Could you check a few things on this model? Use its own coordinates, in mm. Face numbers are marked on the shaded views. Coordinates: 2 decimals unless noted, no trailing zeros. Order: outer loops, then holes, each group sorted by start corner. A loop starts at its lowest first (then second) coordinate and runs counter-clockwise, first axis right, second up. Notation, with made-up numbers: M 60.5,16 L 102.5,16 A32 cw 102.5,52 Z; hole C 7.25,40.5 d9. An arc over 180 degrees is marked long. Write item = value, one per line. Start each with the question number.
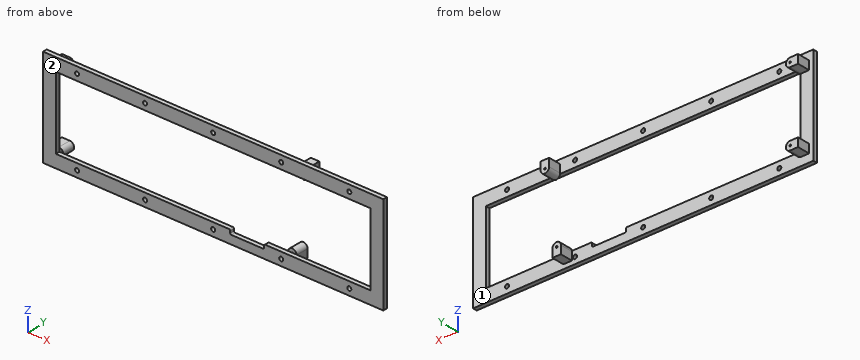
from build123d import *

# Parameters (mm, degrees)
SKETCH1_W           = 254
SKETCH1_H           = 72.69988
SKETCH1_R           = 1.5
BOSS_EXTRUDE1_DEPTH = 3.175
SKETCH1_7_R         = 0.635
BOSS_EXTRUDE2_DEPTH = 9.525


with BuildPart() as part:
    # Sketch1 → Boss-Extrude1 (new body)
    with BuildSketch(Plane(origin=(0, 0, 0), x_dir=(1, 0, 0), z_dir=(0, 1, 0))):
        with Locations((127, 36.34994)):
            Rectangle(SKETCH1_W, SKETCH1_H)
        with Locations(Location((177.8, 67.93738, 0), (0, 0, 270))):
            Circle(SKETCH1_R, mode=Mode.SUBTRACT)
        with Locations(Location((177.8, 4.7625, 0), (0, 0, 90))):
            Circle(SKETCH1_R, mode=Mode.SUBTRACT)
        with Locations(Location((228.6, 67.93738, 0), (0, 0, 270))):
            Circle(SKETCH1_R, mode=Mode.SUBTRACT)
        with Locations(Location((228.6, 4.7625, 0), (0, 0, 90))):
            Circle(SKETCH1_R, mode=Mode.SUBTRACT)
        with Locations(Location((127, 67.93738, 0), (0, 0, 270))):
            Circle(SKETCH1_R, mode=Mode.SUBTRACT)
        with Locations(Location((127, 4.7625, 0), (0, 0, 90))):
            Circle(SKETCH1_R, mode=Mode.SUBTRACT)
        with Locations(Location((25.4, 4.7625, 0), (0, 0, 270))):
            Circle(SKETCH1_R, mode=Mode.SUBTRACT)
        with Locations(Location((76.2, 4.7625, 0), (0, 0, 270))):
            Circle(SKETCH1_R, mode=Mode.SUBTRACT)
        with Locations(Location((25.4, 67.93738, 0), (0, 0, 90))):
            Circle(SKETCH1_R, mode=Mode.SUBTRACT)
        with Locations(Location((76.2, 67.93738, 0), (0, 0, 90))):
            Circle(SKETCH1_R, mode=Mode.SUBTRACT)
        with BuildLine():
            Line((244.475, 63.17488), (244.475, 9.525))
            Line((244.475, 9.525), (9.525, 9.525))
            Line((9.525, 9.525), (9.525, 63.17488))
            Line((9.525, 63.17488), (138.90625, 63.17488))
            ThreePointArc((138.90625, 63.17488), (139.467516008, 63.407363992), (139.7, 63.96863))
            Line((139.7, 63.96863), (139.7, 65.55613))
            ThreePointArc((139.7, 65.55613), (139.932483992, 66.117396008), (140.49375, 66.34988))
            Line((140.49375, 66.34988), (164.30625, 66.34988))
            ThreePointArc((164.30625, 66.34988), (164.867516008, 66.117396008), (165.1, 65.55613))
            Line((165.1, 65.55613), (165.1, 63.96863))
            ThreePointArc((165.1, 63.96863), (165.332483992, 63.407363992), (165.89375, 63.17488))
            Line((165.89375, 63.17488), (244.475, 63.17488))
        make_face(mode=Mode.SUBTRACT)
    extrude(amount=-BOSS_EXTRUDE1_DEPTH)

    # Sketch1_7 → Boss-Extrude2 (add)
    # profile 1 of 4: a face of its own
    with BuildSketch(Plane(origin=(0, 0, 0), x_dir=(1, 0, 0), z_dir=(0, 1, 0))):
        with BuildLine():
            Line((180.1749, 69.52488), (186.5249, 69.52488))
            Line((186.5249, 69.52488), (186.5249, 63.533223536))
            ThreePointArc((186.5249, 63.533223536), (183.3499, 60.358223536), (180.1749, 63.533223536))
            Line((180.1749, 63.533223536), (180.1749, 69.52488))
        make_face()
        with Locations(Location((183.3499, 63.533223536, 0), (0, 0, 325.644879026))):
            Circle(SKETCH1_7_R, mode=Mode.SUBTRACT)
    # profile 2 of 4: a face of its own
    with BuildSketch(Plane(origin=(0, 0, 0), x_dir=(1, 0, 0), z_dir=(0, 1, 0))):
        with BuildLine():
            Line((188.9252, 9.10082), (188.9252, 3.175))
            Line((188.9252, 3.175), (195.2752, 3.175))
            Line((195.2752, 3.175), (195.2752, 9.10082))
            ThreePointArc((195.2752, 9.10082), (192.1002, 12.27582), (188.9252, 9.10082))
        make_face()
        with Locations(Location((192.1002, 9.10082, 0), (0, 0, 41.912890883))):
            Circle(SKETCH1_7_R, mode=Mode.SUBTRACT)
    # profile 3 of 4: a face of its own
    with BuildSketch(Plane(origin=(0, 0, 0), x_dir=(1, 0, 0), z_dir=(0, 1, 0))):
        with BuildLine():
            Line((3.175, 12.27582), (9.10082, 12.27582))
            ThreePointArc((9.10082, 12.27582), (12.27582, 9.10082), (9.10082, 5.92582))
            Line((9.10082, 5.92582), (3.175, 5.92582))
            Line((3.175, 5.92582), (3.175, 12.27582))
        make_face()
        with Locations(Location((9.10082, 9.10082, 0), (0, 0, 48.087109117))):
            Circle(SKETCH1_7_R, mode=Mode.SUBTRACT)
    # profile 4 of 4: a face of its own
    with BuildSketch(Plane(origin=(0, 0, 0), x_dir=(1, 0, 0), z_dir=(0, 1, 0))):
        with BuildLine():
            Line((3.175, 66.708223536), (9.10082, 66.708223536))
            ThreePointArc((9.10082, 66.708223536), (12.27582, 63.533223536), (9.10082, 60.358223536))
            Line((9.10082, 60.358223536), (3.175, 60.358223536))
            Line((3.175, 60.358223536), (3.175, 66.708223536))
        make_face()
        with Locations(Location((9.10082, 63.533223536, 0), (0, 0, 325.644879026))):
            Circle(SKETCH1_7_R, mode=Mode.SUBTRACT)
    extrude(amount=BOSS_EXTRUDE2_DEPTH)


solid = part.part
(1) Will these pins go through, and if not, where does the flat tip stop? P1, Ø5, axis at y = 6.5, z = -7.5, coming from the -X side (3 decimals); P2, Ø7, axis at x = 184, y = 4, coming from the -Z side; P3, Ø3, axis at x = 7, y = 4.5, coming from the +Z side; P4, Ø6, axis at x = 31.5, z = -13, coming from the -Y side.
(2) Please list where these lines run through material, in increasing order: probe 1 along Z at (x, y) = (177.8, -0.65) (1 decimal); probe 2 along X at (y, z) = (-1.75, -54.5) (3 decimals); probe 3 along Y at (x, z) = (102, -66) (3 decimals). Write a range as from..to.
(3) Imagine slicing it at A-A on x = 16. List the corners of the cut face in (y, z) for me (3 decimals).
(4) Imagine slicing it at C-C on z = -16.5. List the corners of the cut face in (x, y) for me (3 decimals).
(5) Thinking about a two-plate mould opening in X: for the marked faces 1 and 2, which applies, released by +X, released by -X, zero draft, split by the parting line, or undercut?
(6) Imagine slicing it at B-B on y = 2. List the corners of the cut face in (x, z) for me (3 decimals).
Response:
q1.P1 = 3.175
q1.P2 = -69.52
q1.P3 = -5.93
q1.P4 = through
q2.probe_1 = -72.7..-69.4, -66.4..-63.2, -9.5..-6.3, -3.3..0
q2.probe_2 = 0..9.525, 244.475..254
q2.probe_3 = -3.175..0
q3.outline = M -3.175,-72.7 L 0,-72.7 L 0,-63.175 L -3.175,-63.175 Z; M -3.175,-9.525 L 0,-9.525 L 0,0 L -3.175,0 Z
q4.outline = M 0,-3.175 L 9.525,-3.175 L 9.525,0 L 0,0 Z; M 244.475,-3.175 L 254,-3.175 L 254,0 L 244.475,0 Z
q5.face_1 = undercut
q5.face_2 = zero draft
q6.outline = M 3.175,-66.708 L 9.101,-66.708 A3.175 ccw 9.101,-60.358 L 3.175,-60.358 Z; M 3.175,-12.276 L 9.101,-12.276 A3.175 ccw 9.101,-5.926 L 3.175,-5.926 Z; M 180.175,-69.525 L 186.525,-69.525 L 186.525,-63.533 A3.175 ccw 180.175,-63.533 Z; M 188.925,-9.101 A3.175 ccw 195.275,-9.101 L 195.275,-3.175 L 188.925,-3.175 Z; hole C 9.101,-63.533 d1.27; hole C 9.101,-9.101 d1.27; hole C 183.35,-63.533 d1.27; hole C 192.1,-9.101 d1.27
